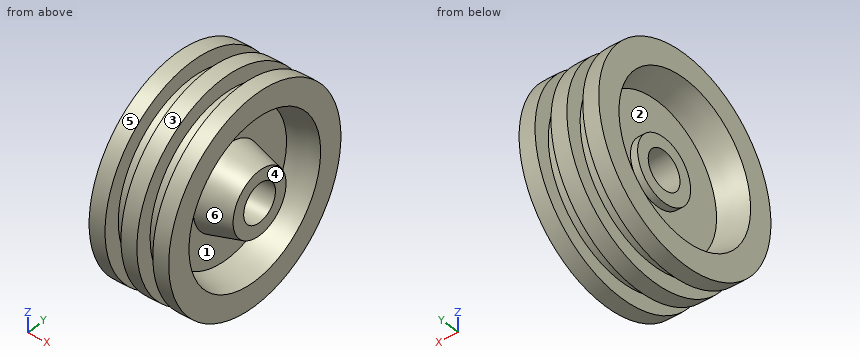
from build123d import *


with BuildPart() as part:
    # Эскиз1 → Повернуть1 (revolve)
    with BuildSketch(Plane.XY, mode=Mode.PRIVATE) as revolve_1_sk:
        Polygon((0, 65), (0, 49.689110868), (17.5, 45), (17.5, 20), (13, 20), (13, 12), (53, 12), (53, 20), (32.5, 25.492958445), (32.5, 45), (50, 49.689110868), (50, 65), (40, 65), (40, 55), (30, 55), (30, 65), (20, 65), (20, 55), (10, 55), (10, 65), align=None)
    revolve(revolve_1_sk.sketch.rotate(Axis((-926.28656243, 0, 0), (1, 0, 0)), 90), axis=Axis((-926.28656243, 0, 0), (1, 0, 0)))


solid = part.part
CAD build for the part. Positions are in the model's coordinates, mm. Face numbers are marked on the shaded views. A direction names the side the tool comes from. Give positions to 0.01 mm unless a question says otherwise; leave off trailing zeros. Write each loop counter-clockwise with the first axis right and the second up, starting at its lowest first coordinate (ties: lowest second). Pieces come first, ordered by that corner, then holes. Notation, with made-up numbers: (43, 6.25) -> (98, 6.25) arc R23 ccw to (98, 43.25) -> close; hole circle Ø5 at (39.5, -32). An arc over 180 degrees is marked (long way). Return JSON: item names as keys, results as strings.
Item 1: Drill centre lines: probe 1 along X at (y, z) = (35, 52.5); probe 2 along Y at (x, z) = (35, 0); probe 3 along Y at (x, z) = (36, 0). Where is each one in solid material? Low to high.
Answer below:
{"probe 1": "x = 0 to 10, 20 to 30, 40 to 50", "probe 2": "y = -55 to -45.67, -24.82 to -12, 12 to 24.82, 45.67 to 55", "probe 3": "y = -55 to -45.94, -24.56 to -12, 12 to 24.56, 45.94 to 55"}
Item 2: Tool access for the marked faces 1, 2 and 3: list every direction of +Z, -Z, +X, -X, +Y, -Y with a clear straight run to the whole face (end or side of a thin tool).
Answer below:
{"face 1": "+X", "face 2": "-X", "face 3": "+X, -X"}
Item 3: Two-plate mould, pull along Y, no slides. Class the marked faces 4, 5 and 6: +Y half, -Y half, draft (parallel to the pull), parting line (faces both ways), or undercut.
Answer below:
{"face 4": "draft", "face 5": "parting line", "face 6": "undercut"}
Item 4: Band-saw the part on A-A (x = 38). List the corners of the cut face in (y, z), then the cut area to 3 significant figures.
Answer below:
{"outline": "circle Ø110 at (0, 0); circle Ø48.04 at (0, 0); hole circle Ø92.95 at (0, 0); hole circle Ø24 at (0, 0)", "area": "4,080 mm2"}
Item 5: Band-saw the part on B-B (x = 4). List the corners of the cut face in (y, z).
Answer below:
{"outline": "circle Ø130 at (0, 0); hole circle Ø97.23 at (0, 0)"}
Item 6: Drop flat-ended pins along their axis: pin 1 (12 mm diameter, centred on y = 22, z = 5, fed in from -X); pin 2 (3 mm diameter, centred on x = 21.5, z = 7.5, fed in from -Y); pin 3 (21.5 mm diameter, centred on y = 0, z = 0, fed in from +X); pin 4 (8 mm diameter, centred on x = 43, z = 40.5, fed in from -Y). Give the stop position or say it passes through.
Answer below:
{"pin 1": "stops at x = 13", "pin 2": "stops at y = -64.72", "pin 3": "passes through", "pin 4": "stops at y = -53.78"}
